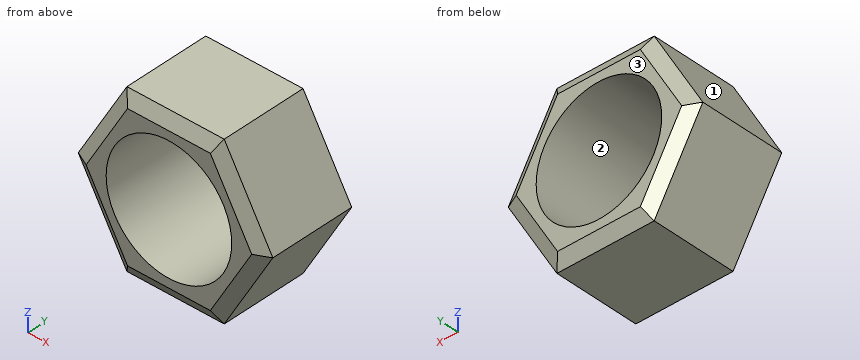
```python
from build123d import *

# Parameters (mm, degrees)
SKETCH_1_R      = 5
EXTRUDE_1_DEPTH = 8
CHAMFER_1_SIZE  = 1
CHAMFER_1_SIZE2 = 0.577350269
CHAMFER_2_SIZE  = 1
CHAMFER_2_SIZE2 = 0.577350269


with BuildPart() as part:
    # Эскиз1 → Бобышка-Вытянуть1 (new body)
    with BuildSketch(Plane(origin=(0, 0, 0), x_dir=(1, 0, 0), z_dir=(0, 1, 0))):
        Polygon((-7.75, 0), (-3.875, -6.711696879), (3.875, -6.711696879), (7.75, 0), (3.875, 6.711696879), (-3.875, 6.711696879), align=None)
        Circle(SKETCH_1_R, mode=Mode.SUBTRACT)
    extrude(amount=EXTRUDE_1_DEPTH)

    # Фаска1
    chamfer_1_edges = [part.edges().sort_by_distance(p)[0] for p in [
        (0, 8, 6.711696879),
        (5.8125, 8, 3.35584844),
        (5.8125, 8, -3.35584844),
        (0, 8, -6.711696879),
        (-5.8125, 8, -3.35584844),
        (-5.8125, 8, 3.35584844),
    ]]
    chamfer_1_side = [part.faces().sort_by_distance(p)[0] for p in [
        (-5.634925192, 8, 3.253325576),
    ]]
    chamfer(chamfer_1_edges, length=CHAMFER_1_SIZE, length2=CHAMFER_1_SIZE2, reference=chamfer_1_side[0])

    # Фаска2
    chamfer_2_edges = [part.edges().sort_by_distance(p)[0] for p in [
        (0, 0, -6.711696879),
        (5.8125, 0, -3.35584844),
        (5.8125, 0, 3.35584844),
        (0, 0, 6.711696879),
        (-5.8125, 0, 3.35584844),
        (-5.8125, 0, -3.35584844),
    ]]
    chamfer_2_side = [part.faces().sort_by_distance(p)[0] for p in [
        (-5.634925192, 0, 3.253325576),
    ]]
    chamfer(chamfer_2_edges, length=CHAMFER_2_SIZE, length2=CHAMFER_2_SIZE2, reference=chamfer_2_side[0])


solid = part.part
```
Geometry: final body of the model. Coordinates: model frame, mm. Face numbers are marked on the shaded views. Coordinates: 2 decimals unless noted, no trailing zeros. Order: outer loops, then holes, each group sorted by start corner. A loop starts at its lowest first (then second) coordinate and runs counter-clockwise, first axis right, second up. Notation, with made-up numbers: M 84,33.25 L 91,33.25 A24 cw 91,57.25 Z; hole C 9,-26.5 d8. An arc over 180 degrees is marked long. Answer in a Markdown table with one row per item. Add a question column.
Q1. Section query A-A on x = 0. Return the cut outline in (y, z).
Q2. Contact query for flat-ended pins moving along their axis: P1, Ø1, axis at x = -5, y = 2, coming from the +Z side; P2, Ø6, axis at x = 2, z = -0.5, coming from the -Y side; P3, Ø1, axis at y = 2, z = 1.5, coming from the -X side. Output: stop coordinate, or through.
Q3. Section query B-B on z = 1.75. Return the cut outline in (x, y), and give its area (3 significant figures).
Q4. Section query C-C on y = 6. Return the cut outline in (x, z) (3 decimals).
Q5. Mould query, pull axis Z, two halves, no side actions, for the marked faces 1, 2 and 3. Classes: released by +Z, released by -Z, zero draft, split by the parting line, or undercut.
Q6. Section query D-D on x = 5.75. Return the cut outline in (y, z), and give its area (3 significant figures).
Q7. Line query: L1, parallel to Z at x = 0, y = 1.5; L2, parallel to X at y = 6.5, z = -3; L3, parallel to Z at x = -1, y = 6.25. Output: solid intervals per line, ascending.
Completed:
| question | item | result |
|---|---|---|
| 1 | outline | M 0,-5.71 L 0.58,-6.71 L 7.42,-6.71 L 8,-5.71 L 8,-5 L 0,-5 Z; M 0,5 L 8,5 L 8,5.71 L 7.42,6.71 L 0.58,6.71 L 0,5.71 Z |
| 2 | P1 | stops at z = 5.63 |
| 2 | P2 | stops at y = 0 |
| 2 | P3 | stops at x = -7.17 |
| 3 | outline | M -6.74,0.58 L -5.58,0 L -4.68,0 L -4.68,8 L -5.58,8 L -6.74,7.42 Z; M 4.68,0 L 5.58,0 L 6.74,0.58 L 6.74,7.42 L 5.58,8 L 4.68,8 Z |
| 3 | area | 31.6 mm2 |
| 4 | outline | M -7.75,0 L -3.875,-6.712 L 3.875,-6.712 L 7.75,0 L 3.875,6.712 L -3.875,6.712 Z; hole C 0,0 d10 |
| 5 | face 1 | released by +Z |
| 5 | face 2 | undercut |
| 5 | face 3 | zero draft |
| 6 | outline | M 0,-1.46 L 0.58,-3.46 L 7.42,-3.46 L 8,-1.46 L 8,1.46 L 7.42,3.46 L 0.58,3.46 L 0,1.46 Z |
| 6 | area | 53.1 mm2 |
| 7 | L1 | z = -6.71 to -5, 5 to 6.71 |
| 7 | L2 | x = -6.02 to -4, 4 to 6.02 |
| 7 | L3 | z = -6.71 to -4.9, 4.9 to 6.71 |
